Autodesk Inventor part; units mm, degrees
ref_plane "YZ Plane" through (0, 0, 0) normal (1, 0, 0) x (0, 1, 0)
ref_plane "XZ Plane" through (0, 0, 0) normal (0, 1, 0) x (-1, 0, 0)
ref_plane "XY Plane" through (0, 0, 0) normal (0, 0, 1) x (1, 0, 0)
sketch "Sketch1" plane through (0, 0, 0) normal (0, 0, 1) x (1, 0, 0)
  circle A0 centre (0, 0) radius 14
  circle A1 centre (0, 0) radius 10.5
  line L0 (14, 0) -> (-14, 0)
  line L1 (-14, 0) -> (-14, -84.5)
  line L2 (-14, -84.5) -> (14, -84.5)
  line L3 (14, -84.5) -> (14, 0)
  dimension "d0" = 28
  dimension "d1" = 21
  dimension "d2" = 84.5
extrude "Extrusion1" add sketch "Sketch1" against normal blind 15 contours L0 A1 A0 | L3 L2 L1 A0 | A0 L0 A1
properties part number "HandSupport"
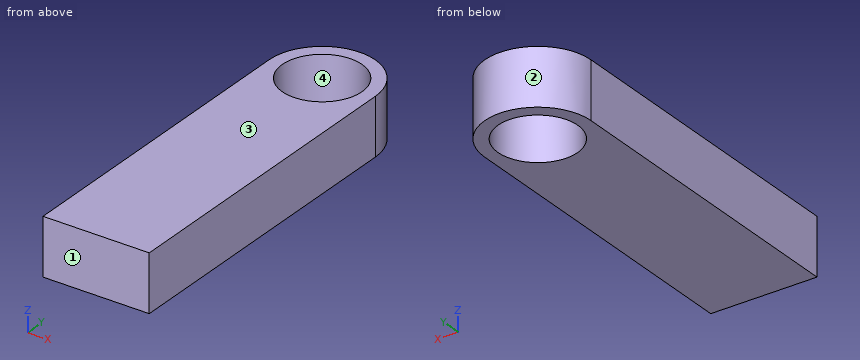
Build history of the part. All positions in model axes, mm. Face numbers are marked on the shaded views. Round coordinates to 2 decimals unless told otherwise and drop trailing zeros. Loops run counter-clockwise (first coordinate to the right, second up) from the corner with the lowest first, then second, coordinate; pieces in that order, holes last.
Item 1: Pin check, flat tip, straight feed: P1, Ø8, axis at x = -9.5, z = -3, coming from the +Y side. Stop position of the tip, or through.
Item 2: Saw through at C-C (z = -4.5). List the corners of the cut face in (x, y), then the cut area to 3 significant figures.
Item 3: Two-plate mould, pull along Y, no slides. Class the marked faces 1, 2, 3 and 4: released by +Y, released by -Y, zero draft, split by the parting line, or undercut.
Item 4: Saw through at D-D (x = -12.25). List the corners of the cut face in (y, z).
Item 5: Saw through at A-A (x = 0). List the corners of the cut face in (y, z).
Item 6: Saw through at B-B (y = 1.5). List the corners of the cut face in (x, z), then the cut area to 3 significant figures.
Item 7: Drill centre lines: line 1 along X through (y, z) = (0, -7.75); line 2 along Y through (x, z) = (0, -10.75); line 3 along Y through (x, z) = (1.75, -12). Where is each one in solid material? Low to high.
Worked answers:
1. P1: stops at y = 12.87
2. outline: (-14, -84.5) - (14, -84.5) - (14, 0) arc R14 ccw to (-14, 0) - close; hole circle Ø21 at (0, 0)
2. area: 2,330 mm2
3. face 1: released by -Y
3. face 2: released by +Y
3. face 3: zero draft
3. face 4: undercut
4. outline: (-84.5, -15) - (6.78, -15) - (6.78, 0) - (-84.5, 0) - close
5. outline: (-84.5, -15) - (-10.5, -15) - (-10.5, 0) - (-84.5, 0) - close; (10.5, -15) - (14, -15) - (14, 0) - (10.5, 0) - close
6. outline: (-13.92, -15) - (-10.39, -15) - (-10.39, 0) - (-13.92, 0) - close; (10.39, -15) - (13.92, -15) - (13.92, 0) - (10.39, 0) - close
6. area: 106 mm2
7. line 1: x = -14 to -10.5, 10.5 to 14
7. line 2: y = -84.5 to -10.5, 10.5 to 14
7. line 3: y = -84.5 to -10.35, 10.35 to 13.89
